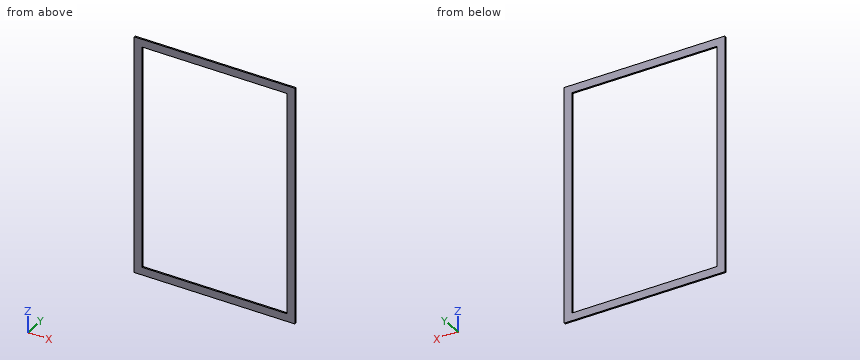
Autodesk Inventor part; units mm, degrees
ref_plane "YZ Plane" through (0, 0, 0) normal (1, 0, 0) x (0, 1, 0)
ref_plane "XZ Plane" through (0, 0, 0) normal (0, 1, 0) x (-1, 0, 0)
ref_plane "XY Plane" through (0, 0, 0) normal (0, 0, 1) x (1, 0, 0)
sketch "Boceto1" plane through (0, 0, 0) normal (0, 1, 0) x (-1, 0, 0)
  line L0 (0, 0) -> (280, 0)
  line L1 (280, 0) -> (280, -430)
  line L2 (280, -430) -> (0, -430)
  line L3 (0, -430) -> (0, 0)
  line L4 (0, 15) -> (295, 15)
  line L5 (295, 15) -> (295, -445)
  line L6 (295, -445) -> (-15, -445)
  line L7 (-15, -445) -> (-15, 15)
  line L8 (-15, 15) -> (0, 15)
  dimension "d0" = 280
  dimension "d1" = 430
  dimension "d2" = 15
  dimension "d3" = 295
  dimension "d4" = 460
  dimension "d5" = 310
extrude "Extrusión1" add sketch "Boceto1" along normal blind 3
properties part number "Marco molde"
Can you work these out from the model? Positions are in its coordinate system, mm. Give positions to 0.01 mm unless a question says otherwise; leave off trailing zeros. Order: outer loops, then holes, each group sorted by start corner. A loop starts at its lowest first (then second) coordinate and runs counter-clockwise, first axis right, second up. Notation, with made-up numbers: M 29,59 L 44,59 A18 cw 44,91 Z; hole C -7.75,45 d10. An arc over 180 degrees is marked long. Use one line per item in the form item = value. Start each with the question number.
Item 1: If I drill on line 1 along Z through (x, y) = (-59, 1.05); line 2 along X through (y, z) = (1.15, -331), over which ranges is the centre line in solid material (lowest first)?
Item 2: If we section it at B-B (z = -241.5): Write out the boundary of the cut face in (x, y).
Item 3: If we section it at A-A (x = -136.5): Write out the boundary of the cut face in (y, z), then the cut area to 3 significant figures.
Item 4: If we section it at C-C (y = 0.9): Write out the boundary of the cut face in (x, z), then the cut area to 3 significant figures.
Outcome:
q1.line_1 = -445 to -430, 0 to 15
q1.line_2 = -295 to -280, 0 to 15
q2.outline = M -295,0 L -280,0 L -280,3 L -295,3 Z; M 0,0 L 15,0 L 15,3 L 0,3 Z
q3.outline = M 0,-445 L 3,-445 L 3,-430 L 0,-430 Z; M 0,0 L 3,0 L 3,15 L 0,15 Z
q3.area = 90.0 mm2
q4.outline = M -295,-445 L 15,-445 L 15,15 L -295,15 Z; hole M -280,-430 L 0,-430 L 0,0 L -280,0 Z
q4.area = 22,200 mm2
